from build123d import *

# Parameters (mm, degrees)
F0_R      = 40
F2_R      = 55
F3_W      = 11
F3_H      = 10.5
F5_DEPTH  = 15
F7_W      = 51.318744
F7_H      = 15
F8_DEPTH  = 5
F10_DEPTH = 25


with BuildPart() as f4:
    # F0 (on Top) → F4 section 0
    with BuildSketch(Plane.XY):
        Circle(F0_R)
    # F2 (on offset) → F4 section 1
    with BuildSketch(Plane.XY.offset(-30)):
        Circle(F2_R)
    loft()

    # F3 (on Top) → F5 (cut)
    with BuildSketch(Plane.XY):
        Polygon((0, 0), (0, 10.5), (-31, 10.5), (-31, -10.5), (11, -10.5), (11, 0), align=None)
        with Locations((5.5, 5.25)):
            Rectangle(F3_W, F3_H)
    extrude(amount=-F5_DEPTH, mode=Mode.SUBTRACT)

    # F7 (on face) → F8 (cut)
    with BuildSketch(Plane(origin=(0, 0, -30), x_dir=(1, 0, 0), z_dir=(0, 0, -1))):
        with Locations((30.659372, 0)):
            Rectangle(F7_W, F7_H)
    extrude(amount=-F8_DEPTH, mode=Mode.SUBTRACT)

    # F9 (on face) → F10 (cut)
    with BuildSketch(Plane.XY):
        Polygon((11, 5), (11, 0), (11, -5), (23.5, -5), (23.5, 5), align=None)
    extrude(amount=-F10_DEPTH, mode=Mode.SUBTRACT)


solid = f4.part
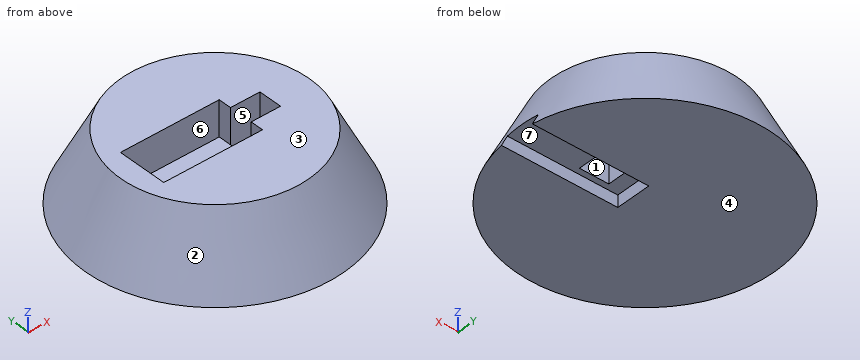
Geometry: final body of the model. Coordinates: model frame, mm. Face numbers are marked on the shaded views. A direction names the side the tool comes from. Give positions to 0.01 mm unless a question says otherwise; leave off trailing zeros. Loops run counter-clockwise (first coordinate to the right, second up) from the corner with the lowest first, then second, coordinate; pieces in that order, holes last. Notation, with made-up numbers: M 20.5,-11 L 56.5,-11 A34 ccw 56.5,27 Z; hole C -13,-37.75 d4. An arc over 180 degrees is marked long. Put each result on its own line as item: value.
1) Material intervals for L1, parallel to Y at x = -26, z = -3; L2, parallel to Y at x = 11.5, z = -11; L3, parallel to Z at x = -25, y = 10, sorted ascending. Write a range as from..to.
Computed values:
L1: y = -32.35..-10.5, 10.5..32.35
L2: y = -44.02..-5, 5..44.02
L3: z = -30..-15
2) Reachability of the marked faces 4, 5, 6 and 7 from +Z, -Z, +X, -X, +Y, -Y: full face, straight path, thin tool, end or side. Return the list, or none.
Computed values:
face 4: -Z, +X, -X, +Y, -Y
face 5: +Z, -Z
face 6: +Z
face 7: -Z, +X
3) Cut plane A-A, the plane z = -5.5. Return the cut outline in (x, y).
Computed values:
outline: C 0,0 d85.5; hole M -31,-10.5 L 11,-10.5 L 11,-5 L 23.5,-5 L 23.5,5 L 11,5 L 11,10.5 L -31,10.5 Z
4) Cut plane B-B, the plane x = 0. Return the cut outline in (y, z).
Computed values:
outline: M -55,-30 L 55,-30 L 40,0 L 10.5,0 L 10.5,-15 L -10.5,-15 L -10.5,0 L -40,0 Z
5) Cut plane C-C, the plane z = -18. Return the cut outline in (x, y).
Computed values:
outline: C 0,0 d98; hole M 11,-5 L 23.5,-5 L 23.5,5 L 11,5 Z
6) First-contact query: P1, Ø7.5, axis at x = -16.5, z = -7.5, coming from the -Y side; P2, Ø4, axis at x = 31, z = -26.5, coming from the +Y side; P3, Ø5.5, axis at x = 29, z = -26.5, coming from the -Y side; P4, Ø3, axis at x = -30.5, y = 17.5, coming from the +Z side. Flat tips, straight axial feed; report the tip coordinate or a pass-through.
Computed values:
P1: stops at y = -42.95
P2: stops at y = 45.12
P3: stops at y = -46.99
P4: stops at z = 0
7) Mould query, pull axis Y, two halves, no side actions, for the marked faces 1, 2 and 3. Classes: released by +Y, released by -Y, zero draft, split by the parting line, or undercut.
Computed values:
face 1: undercut
face 2: split by the parting line
face 3: zero draft
